from build123d import *

# Parameters (mm, degrees)
SKETCH1_W           = 15
SKETCH1_H           = 15
BOSS_EXTRUDE1_DEPTH = 5
CUT_EXTRUDE1_DEPTH  = 18.5
SKETCH3_R           = 2
CUT_EXTRUDE2_DEPTH  = 12.7260394
SKETCH4_W           = 9
SKETCH4_H           = 7
CUT_EXTRUDE4_DEPTH  = 3


with BuildPart() as part:
    # Sketch1 → Boss-Extrude1 (new body)
    with BuildSketch(Plane.XY):
        Rectangle(SKETCH1_W, SKETCH1_H)
    extrude(amount=BOSS_EXTRUDE1_DEPTH)

    # Sketch2 → Cut-Extrude1 (cut, through all)
    with BuildSketch(Plane.ZY.offset(7.5)):
        Polygon((1, 7.5), (5, 3.5), (5, 7.5), align=None)
        Polygon((1, -7.5), (5, -3.5), (5, -7.5), align=None)
    extrude(amount=-CUT_EXTRUDE1_DEPTH, mode=Mode.SUBTRACT)

    # Sketch3 → Cut-Extrude2 (cut, through all)
    with BuildSketch(Plane.XY.offset(5)):
        Circle(SKETCH3_R)
    extrude(amount=-CUT_EXTRUDE2_DEPTH, mode=Mode.SUBTRACT)

    # Sketch4 → Cut-Extrude4 (cut)
    with BuildSketch(Plane.XY.offset(5)):
        Rectangle(SKETCH4_W, SKETCH4_H)
    extrude(amount=-CUT_EXTRUDE4_DEPTH, mode=Mode.SUBTRACT)


solid = part.part
The listing builds one solid part. Answer for the finished solid, in the listing's coordinates (mm). A direction names the side the tool comes from. Give positions to 0.01 mm unless a question says otherwise; leave off trailing zeros. Loops run counter-clockwise (first coordinate to the right, second up) from the corner with the lowest first, then second, coordinate; pieces in that order, holes last. Notation, with made-up numbers: M 41.5,-7.5 L 74.5,-7.5 A28 cw 74.5,21.5 Z; hole C 78,2 d7. An arc over 180 degrees is marked long. Answer as CSV lines item,"result".
Item 1: Straight lines are drawn through the part: line 1 along X through (y, z) = (3, 4.8); line 2 along Y through (x, z) = (0, 0.85); line 3 along Z through (x, y) = (-5.5, 4). For each, find the intervals that lie inside material, in ascending order. Write a range as [from, to].
Values follow:
line 1,"x = [-7.5, -4.5], [4.5, 7.5]"
line 2,"y = [-7.5, -2], [2, 7.5]"
line 3,"z = [0, 4.5]"
Item 2: The part is cut by section B-B (z = 2.6). Give the vertices of the cut face in (x, y).
Values follow:
outline,"M -7.5,-5.9 L 7.5,-5.9 L 7.5,5.9 L -7.5,5.9 Z; hole M -4.5,-3.5 L 4.5,-3.5 L 4.5,3.5 L -4.5,3.5 Z"
Item 3: The part is cut by section A-A (y = 0). Give the vertices of the cut face in (x, z).
Values follow:
outline,"M -7.5,0 L -2,0 L -2,2 L -4.5,2 L -4.5,5 L -7.5,5 Z; M 2,0 L 7.5,0 L 7.5,5 L 4.5,5 L 4.5,2 L 2,2 Z"
Item 4: The mould has two halves that part along X. Classify faces 1 (the flat face through (-4.5, 0, 4)), 2 (the flat face through (-7.5, 0, 2)), 3 (the flat face through (7.5, 0, 2)), 4 (the flat face through (6, 0, 5)): released by +X, released by -X, zero draft, split by the parting line, or undercut.
Values follow:
face 1,"undercut"
face 2,"released by -X"
face 3,"released by +X"
face 4,"zero draft"
Item 5: The part is cut by section D-D (x = 3). Give the vertices of the cut face in (y, z).
Values follow:
outline,"M -7.5,0 L 7.5,0 L 7.5,1 L 3.5,5 L 3.5,2 L -3.5,2 L -3.5,5 L -7.5,1 Z"
Item 6: Given pin 1 Ø2 at (x, y) = (5.5, 5) entering from +Z; pin 2 Ø5.5 at (x, y) = (0, 0.5) entering from +Z; pin 3 Ø0.9 at (x, z) = (-1.5, 4) entering from +Y, each flat-ended and moving along its own axis, determine where each tip first touches the part or whether it passes through.
Values follow:
pin 1,"stops at z = 4.5"
pin 2,"stops at z = 2"
pin 3,"stops at y = 4.95"
Item 7: Which of the six approach directions +Z, -Z, +X, -X, +Y, -Y give full straight-line access (tool end or side, diameter ignored) to faces 5 (the flat face through (-6, 0, 5)), 6 (the flat face through (0, 3.5, 4))?
Values follow:
face 5,"+Z, +X, -X, +Y, -Y"
face 6,"+Z"
Item 8: The part is cut by section C-C (x = 0). Give the vertices of the cut face in (y, z).
Values follow:
outline,"M -7.5,0 L -2,0 L -2,2 L -3.5,2 L -3.5,5 L -7.5,1 Z; M 2,0 L 7.5,0 L 7.5,1 L 3.5,5 L 3.5,2 L 2,2 Z"
